from build123d import *


with BuildPart() as part:
    # Croquis1 → Revolución1 (revolve)
    with BuildSketch(Plane.XY):
        with BuildLine():
            Line((0, 120), (0, 0))
            Line((0, 0), (-1.629604709, 0))
            Line((-1.629604709, 0), (-1.629604709, 33.329604709))
            Line((-1.629604709, 33.329604709), (-1.7, 33.4))
            Line((-1.7, 33.4), (-1.7, 117.7))
            Line((-1.7, 117.7), (-3.35, 117.7))
            Line((-3.35, 117.7), (-3.35, 119))
            ThreePointArc((-3.35, 119), (-3.057106781, 119.707106781), (-2.35, 120))
            Line((-2.35, 120), (0, 120))
        make_face()
    revolve(axis=Axis((0, 120, 0), (0, -1, 0)))


solid = part.part
Verification items for the finished model (mm, model axes). A direction names the side the tool comes from. Give positions to 0.01 mm unless a question says otherwise; leave off trailing zeros. Loops run counter-clockwise (first coordinate to the right, second up) from the corner with the lowest first, then second, coordinate; pieces in that order, holes last.
1) Sectioned sample at B-B, the plane z = 0. Enter the section's corners in (x, y), then the cut area to 3 significant figures.
2) Sectioned sample at D-D, the plane y = 45.5. Enter the section's corners in (x, z).
3) Set-up check for faces 1 (the flat face through (0, 120, 0)), 2 (the cylindrical face through (0.37, 76.14, 1.66)): record each of +Z, -Z, +X, -X, +Y, -Y from which the full face is reachable in a straight line by a thin tool's end or side.
4) Sectioned sample at A-A, the plane x = 0. Enter the section's corners in (y, z), then the cut area to 3 significant figures.
5) Sectioned sample at C-C, the plane y = 30.5. Enter the section's corners in (x, z).
6) Depth check by flat-ended pin: pin 1 Ø1 at (x, z) = (2, 2.5) entering from +Y; pin 2 Ø4 at (y, z) = (73.5, -2) entering from -X; pin 3 Ø1 at (x, y) = (1.5, 54) entering from +Z. Enter the tip coordinate at first touch or a pass-through.
7) Thickness scan on line 1 along Y through (x, z) = (-1.75, 1.25); line 2 along Z through (x, y) = (-0.5, 48.5); line 3 along Z through (x, y) = (-0.25, 102.5). Record the ranges inside material, lowest first.
Answers:
1. outline: (-3.35, 117.7) - (-1.7, 117.7) - (-1.7, 33.4) - (-1.63, 33.33) - (-1.63, 0) - (1.63, 0) - (1.63, 33.33) - (1.7, 33.4) - (1.7, 117.7) - (3.35, 117.7) - (3.35, 119) arc R1 ccw to (2.35, 120) - (-2.35, 120) arc R1 ccw to (-3.35, 119) - close
1. area: 410 mm2
2. outline: circle Ø3.4 at (0, 0)
3. face 1: +Z, -Z, +X, -X, +Y
3. face 2: -Y
4. outline: (0, -1.63) - (33.33, -1.63) - (33.4, -1.7) - (117.7, -1.7) - (117.7, -3.35) - (119, -3.35) arc R1 ccw to (120, -2.35) - (120, 2.35) arc R1 ccw to (119, 3.35) - (117.7, 3.35) - (117.7, 1.7) - (33.4, 1.7) - (33.33, 1.63) - (0, 1.63) - close
4. area: 410 mm2
5. outline: circle Ø3.26 at (0, 0)
6. pin 1: stops at y = 119.94
6. pin 2: stops at x = -1.7
6. pin 3: stops at z = 1.37
7. line 1: y = 117.7 to 120
7. line 2: z = -1.62 to 1.62
7. line 3: z = -1.68 to 1.68
